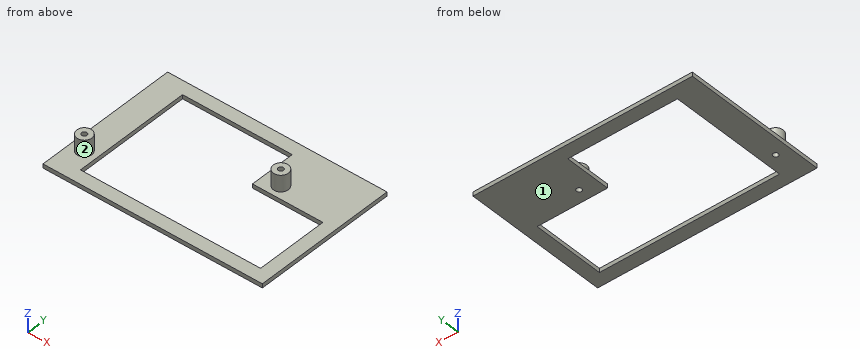
from build123d import *

# Parameters (mm, degrees)
F0_W     = 85.09
F0_H     = 56.134
F1_DEPTH = 1.5875
F2_R     = 2.921
F2_R_2   = 1.016
F3_DEPTH = 6.35
F4_DEPTH = 6.35
F5_W     = 32.385
F5_H     = 22.987
F5_W_2   = 27.305
F5_H_2   = 5.08
F6_DEPTH = 6.35


# Not quite as in the source:
# - a feature names something its author has since deleted; it is built from what else it names


with BuildPart() as f1:
    # F0 (on Top) → F1 (new body)
    with BuildSketch(Plane.XY):
        Rectangle(F0_W, F0_H)
    extrude(amount=F1_DEPTH)

    # F2 (on face) → F3 (join)
    with BuildSketch(Plane.XY.offset(1.5875)):
        with Locations((17.018, 9.906)):
            Circle(F2_R)
        with Locations((17.018, 9.906)):
            Circle(F2_R_2, mode=Mode.SUBTRACT)
        with Locations((-37.338, -15.494)):
            Circle(F2_R)
        with Locations((-37.338, -15.494)):
            Circle(F2_R_2, mode=Mode.SUBTRACT)
    extrude(amount=F3_DEPTH)

    # F2 (on face) → F4 (cut)
    with BuildSketch(Plane.XY.offset(1.5875)):
        with Locations((-37.338, -15.494)):
            Circle(F2_R_2)
        with Locations((17.018, 9.906)):
            Circle(F2_R_2)
    extrude(amount=-F4_DEPTH, mode=Mode.SUBTRACT)

    # F5 (on face) → F6 (cut)
    with BuildSketch(Plane.XY.offset(1.5875)):
        with Locations((-16.1925, 11.4935)):
            Rectangle(F5_W, F5_H)
        Polygon((0, 22.987), (0, 0), (10.16, 0), (10.16, 5.08), (10.16, 22.987), align=None)
        with Locations((23.8125, 2.54)):
            Rectangle(F5_W_2, F5_H_2)
        Polygon((10.16, 0), (0, 0), (0, -22.987), (37.465, -22.987), (37.465, 0), align=None)
        with Locations((-16.1925, -11.4935)):
            Rectangle(F5_W, F5_H)
    extrude(amount=-F6_DEPTH, mode=Mode.SUBTRACT)


solid = f1.part
Source: CAD feature listing. Evaluate the final solid. Frame: model axes, mm. Face numbers are marked on the shaded views. A direction names the side the tool comes from. Coordinates: 2 decimals unless noted, no trailing zeros. Write each loop counter-clockwise with the first axis right and the second up, starting at its lowest first coordinate (ties: lowest second). Pieces come first, ordered by that corner, then holes. Notation, with made-up numbers: M -5.75,-16 L 29.25,-16 A29 ccw 29.25,11 Z; hole C 63.5,15.25 d7. An arc over 180 degrees is marked long. Use a Markdown table: item, result.
1) Section A-A, the plane y = 15. Output: boundary loops of the cut face in (x, z) (1 decimal).
Conclusion:
| item | result |
|---|---|
| outline | M -42.5,0 L -32.4,0 L -32.4,1.6 L -42.5,1.6 Z; M 10.2,0 L 42.5,0 L 42.5,1.6 L 10.2,1.6 Z |
2) Section C-C, the plane z = 3.25. Output: boundary loops of the cut face in (x, y).
Conclusion:
| item | result |
|---|---|
| outline | C -37.34,-15.49 d5.84; C 17.02,9.91 d5.84; hole C -37.34,-15.49 d2.03; hole C 17.02,9.91 d2.03 |
3) Section B-B, the plane x = -21. Output: boundary loops of the cut face in (y, z), then the cut area to 3 significant figures.
Conclusion:
| item | result |
|---|---|
| outline | M -28.07,0 L -22.99,0 L -22.99,1.59 L -28.07,1.59 Z; M 22.99,0 L 28.07,0 L 28.07,1.59 L 22.99,1.59 Z |
| area | 16.1 mm^2 |
4) First-contact query: pin 1 Ø3.5 at (x, y) = (-37.338, -15.494) entering from -Z; pin 2 Ø10 at (x, y) = (-28.5, -18) entering from +Z. Flat tips, straight axial feed; report the tip coordinate or a pass-through.
Conclusion:
| item | result |
|---|---|
| pin 1 | stops at z = 0 |
| pin 2 | stops at z = 1.59 |
5) Reachability of the marked faces 1 and 2 from +Z, -Z, +X, -X, +Y, -Y: full face, straight path, thin tool, end or side. Return the list, or none.
Conclusion:
| item | result |
|---|---|
| face 1 | -Z, +X, -X, +Y, -Y |
| face 2 | +Z |
6) Ray query, L1, parallel to Y at x = 6.5, z = 1; L2, parallel to X at y = 2, z = 0.75 (3 decimals); L3, parallel to X at y = 14, z = 0.5 (3 decimals). Return the intervals inside material, ascending.
Conclusion:
| item | result |
|---|---|
| L1 | y = -28.07 to -22.99, 22.99 to 28.07 |
| L2 | x = -42.545 to -32.385, 37.465 to 42.545 |
| L3 | x = -42.545 to -32.385, 10.16 to 42.545 |
